```python
from build123d import *

# Parameters (mm, degrees)
F0_W     = 160
F0_H     = 40
F1_DEPTH = 5
F2_R     = 16
F3_DEPTH = 5
F5_DEPTH = 2.5


with BuildPart() as f1:
    # F0 (on Top) → F1 (new body)
    with BuildSketch(Plane.XY):
        with Locations((12.406252, 38.980732)):
            Rectangle(F0_W, F0_H)
    extrude(amount=F1_DEPTH)

    # F2 (on face) → F3 (cut)
    with BuildSketch(Plane.XY.offset(5)):
        with Locations((-47.593748, 38.980732)):
            Circle(F2_R)
    extrude(amount=-F3_DEPTH, mode=Mode.SUBTRACT)

    # F4 (on face) → F5 (cut)
    with BuildSketch(Plane.XY.offset(5)):
        Polygon((-53.593748, 20.980732), (-61.593748, 20.980732), (-59.593748, 18.980732), (-55.593748, 18.980732), align=None)
        Polygon((-33.593748, 20.980732), (-41.593748, 20.980732), (-39.593748, 18.980732), (-35.593748, 18.980732), align=None)
        Polygon((-13.593748, 20.980732), (-21.593748, 20.980732), (-19.593748, 18.980732), (-15.593748, 18.980732), align=None)
        Polygon((6.406252, 20.980732), (-1.593748, 20.980732), (0.406252, 18.980732), (4.406252, 18.980732), align=None)
        Polygon((26.406252, 20.980732), (18.406252, 20.980732), (20.406252, 18.980732), (24.406252, 18.980732), align=None)
        Polygon((44.406252, 18.980732), (46.406252, 20.980732), (38.406252, 20.980732), (40.406252, 18.980732), align=None)
        Polygon((64.406252, 18.980732), (66.406252, 20.980732), (58.406252, 20.980732), (60.406252, 18.980732), align=None)
        Polygon((84.406252, 18.980732), (86.406252, 20.980732), (78.406252, 20.980732), (80.406252, 18.980732), align=None)
    extrude(amount=-F5_DEPTH, mode=Mode.SUBTRACT)


solid = f1.part
```
Here's how the part is built. I have some questions about the finished solid (model axes, mm). Coordinates: 2 decimals unless noted, no trailing zeros. Write each loop counter-clockwise with the first axis right and the second up, starting at its lowest first coordinate (ties: lowest second). Pieces come first, ordered by that corner, then holes. Notation, with made-up numbers: (50.25, 39.5) -> (101.25, 39.5) arc R26 cw to (101.25, 57.5) -> close; hole circle Ø11 at (31, -30.5). An arc over 180 degrees is marked (long way). Use a Markdown table: item, result. Add a question column.
(1) We'd pull the mould along Y, two halves only. Please class faces 1 (the flat face through (11, 58.981, 2)), 2 (the flat face through (22, 20.981, 4)), 3 (the flat face through (62, 20.981, 4)), 4 (the flat face through (29, 39, 0)): +Y half, -Y half, draft (parallel to the pull), parting line (faces both ways), or undercut.
(2) If we section it at B-B, the plane y = 25.5: Write out the boundary of the cut face in (x, z), and give its area (3 significant figures).
(3) Please list where these lines run through material, in increasing order: line 1 (Y direction, x = -34.5, z = 4.2); line 2 (X direction, y = 39, z = 4.7); line 3 (Y direction, x = 42, z = 2.8).
(4) If we section it at C-C, the plane z = 1: Write out the boundary of the cut face in (x, y).
(5) I'm going to push flat-ended pins straight in: P1, Ø0.8, axis at x = -37, z = 4, coming from the -Y side; P2, Ø1.6, axis at x = 1, y = 20, coming from the +Z side; P3, Ø10, axis at x = 68, y = 25.5, coming from the -Z side. Where does each tip first touch, or does it pass through?
(6) If we section it at A-A, the plane y = 33: Write out the boundary of the cut face in (x, z).
Outcome:
| question | item | result |
|---|---|---|
| 1 | face 1 | +Y half |
| 1 | face 2 | undercut |
| 1 | face 3 | undercut |
| 1 | face 4 | draft |
| 2 | outline | (-67.59, 0) -> (-56.21, 0) -> (-56.21, 5) -> (-67.59, 5) -> close; (-38.98, 0) -> (92.41, 0) -> (92.41, 5) -> (-38.98, 5) -> close |
| 2 | area | 714 mm^2 |
| 3 | line 1 | y = 18.98 to 20.07, 20.98 to 29.79, 48.18 to 58.98 |
| 3 | line 2 | x = -67.59 to -63.59, -31.59 to 92.41 |
| 3 | line 3 | y = 20.98 to 58.98 |
| 4 | outline | (-67.59, 18.98) -> (92.41, 18.98) -> (92.41, 58.98) -> (-67.59, 58.98) -> close; hole circle Ø32 at (-47.59, 38.98) |
| 5 | P1 | stops at y = 20.98 |
| 5 | P2 | stops at z = 2.5 |
| 5 | P3 | stops at z = 0 |
| 6 | outline | (-67.59, 0) -> (-62.43, 0) -> (-62.43, 5) -> (-67.59, 5) -> close; (-32.75, 0) -> (92.41, 0) -> (92.41, 5) -> (-32.75, 5) -> close |
